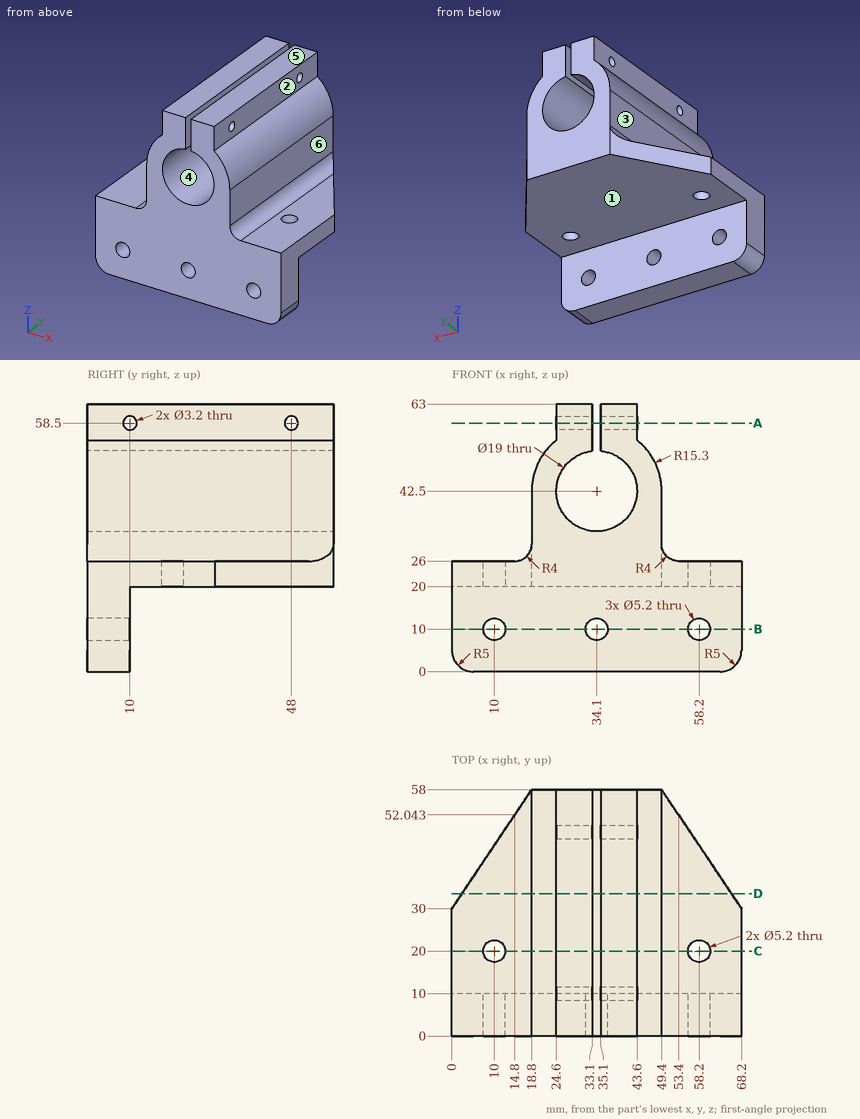
Verification items for this drawing (mm, ordinates from the low corner). A direction names the side the tool comes from. Round coordinates to 2 decimals unless told otherwise and drop trailing zeros. Order: outer loops, then holes, each group sorted by start corner. A loop starts at its lowest first (then second) coordinate and runs counter-clockwise, first axis right, second up. Notation, with made-up numbers: (-9.75, 86) -> (26.25, 86) arc R16 ccw to (26.25, 116) -> close; hole circle Ø3 at (80.25, 89). An arc over 180 degrees is marked (long way). Use one line per item in the form item = value.
1. Scan lines: line 1 along Y through (x, z) = (39.75, 58.5); line 2 along X through (y, z) = (2.75, 10); line 3 along X through (y, z) = (41, 43). Record each from-to range of solid material in increasing order. Write a range as from..to.
Working result:
line_1 = 0..8.4, 11.6..46.4, 49.6..58
line_2 = 0..7.4, 12.6..31.5, 36.7..55.6, 60.8..68.2
line_3 = 18.81..24.61, 43.59..49.39
2. Go/stop test with flat-tipped pins: pin 1 (6 mm diameter, centred on y = 28, z = 35, fed in from -X); pin 2 (10 mm diameter, centred on x = 47.5, z = 8.5, fed in from +Y); pin 3 (5 mm diameter, centred on x = 27, y = 15, fed in from -Z); pin 4 (7 mm diameter, centred on x = 10, z = 10, fed in from -Y). Record where each tip stops, or that it passes through.
Working result:
pin_1 = 18.8
pin_2 = 10
pin_3 = 20
pin_4 = 0
3. Set-up check for the marked faces 1, 2 and 3: record each of +Z, -Z, +X, -X, +Y, -Y from which the full face is reachable in a straight line by a thin tool's end or side.
Working result:
face_1 = -Z, +X, -X, +Y
face_2 = +Z, +X, +Y, -Y
face_3 = +Z, -X, +Y, -Y
4. Cross-section at B-B, the plane z = 10. Enter the section's corners in (x, y), plus the area to 3 significant figures.
Working result:
outline = (0, 0) -> (7.4, 0) -> (7.4, 10) -> (0, 10) -> close; (12.6, 0) -> (31.5, 0) -> (31.5, 10) -> (12.6, 10) -> close; (36.7, 0) -> (55.6, 0) -> (55.6, 10) -> (36.7, 10) -> close; (60.8, 0) -> (68.2, 0) -> (68.2, 10) -> (60.8, 10) -> close
area = 526 mm^2
5. Mould release check, pull along Z, two halves, no side actions. Record for the marked faces 4, 5 and 6: pulls with the +Z half, pulls with the -Z half, needs draft (parallel to the pull), parting line crosses it, or undercut.
Working result:
face_4 = undercut
face_5 = pulls with the +Z half
face_6 = needs draft
6. Cross-section at A-A, the plane z = 58.5. Enter the section's corners in (x, y).
Working result:
outline = (24.6, 0) -> (33.1, 0) -> (33.1, 8.4) -> (24.6, 8.4) -> close; (24.6, 11.6) -> (33.1, 11.6) -> (33.1, 46.4) -> (24.6, 46.4) -> close; (24.6, 49.6) -> (33.1, 49.6) -> (33.1, 58) -> (24.6, 58) -> close; (35.1, 0) -> (43.6, 0) -> (43.6, 8.4) -> (35.1, 8.4) -> close; (35.1, 11.6) -> (43.6, 11.6) -> (43.6, 46.4) -> (35.1, 46.4) -> close; (35.1, 49.6) -> (43.6, 49.6) -> (43.6, 58) -> (35.1, 58) -> close
7. Cross-section at D-D, the plane y = 33.5. Enter the section's corners in (x, z), plus the area to 3 significant figures.
Working result:
outline = (2.35, 20) -> (65.85, 20) -> (65.85, 26) -> (53.4, 26) arc R4 cw to (49.4, 30) -> (49.4, 42.5) arc R15.3 ccw to (43.6, 54.49) -> (43.6, 63) -> (35.1, 63) -> (35.1, 51.95) arc R9.5 cw (long way) to (33.1, 51.95) -> (33.1, 63) -> (24.6, 63) -> (24.6, 54.49) arc R15.3 ccw to (18.8, 42.5) -> (18.8, 30) arc R4 cw to (14.8, 26) -> (2.35, 26) -> close
area = 1,070 mm^2
8. Cross-section at C-C, the plane y = 20. Enter the section's corners in (x, z).
Working result:
outline = (0, 20) -> (7.4, 20) -> (7.4, 26) -> (0, 26) -> close; (12.6, 20) -> (55.6, 20) -> (55.6, 26) -> (53.4, 26) arc R4 cw to (49.4, 30) -> (49.4, 42.5) arc R15.3 ccw to (43.6, 54.49) -> (43.6, 63) -> (35.1, 63) -> (35.1, 51.95) arc R9.5 cw (long way) to (33.1, 51.95) -> (33.1, 63) -> (24.6, 63) -> (24.6, 54.49) arc R15.3 ccw to (18.8, 42.5) -> (18.8, 30) arc R4 cw to (14.8, 26) -> (12.6, 26) -> close; (60.8, 20) -> (68.2, 20) -> (68.2, 26) -> (60.8, 26) -> close
